```python
from build123d import *

# Parameters (mm, degrees)
BOSS_EXTRUDE1_DEPTH = 1.5
SKETCH2_W           = 77.5
SKETCH2_H           = 28.5
SKETCH2_W_2         = 74.5
SKETCH2_H_2         = 25.5
BOSS_EXTRUDE2_DEPTH = 1.5


with BuildPart() as part:
    # Sketch1 → Boss-Extrude1 (new body)
    with BuildSketch(Plane(origin=(0, 0, 0), x_dir=(1, 0, 0), z_dir=(0, 1, 0))):
        with BuildLine():
            Line((-76.546897521, -86.290788706), (-153.546897521, -86.290788706))
            ThreePointArc((-153.546897521, -86.290788706), (-154.961111084, -85.705002268), (-155.546897521, -84.290788706))
            Line((-155.546897521, -84.290788706), (-155.546897521, -56.290788706))
            ThreePointArc((-155.546897521, -56.290788706), (-154.961111084, -54.876575144), (-153.546897521, -54.290788706))
            Line((-153.546897521, -54.290788706), (-76.546897521, -54.290788706))
            ThreePointArc((-76.546897521, -54.290788706), (-75.132683959, -54.876575144), (-74.546897521, -56.290788706))
            Line((-74.546897521, -56.290788706), (-74.546897521, -84.290788706))
            ThreePointArc((-74.546897521, -84.290788706), (-75.132683959, -85.705002268), (-76.546897521, -86.290788706))
        make_face()
    extrude(amount=BOSS_EXTRUDE1_DEPTH)

    # Sketch2 → Boss-Extrude2 (add)
    with BuildSketch(Plane(origin=(0, 1.5, 0), x_dir=(1, 0, 0), z_dir=(0, 1, 0))):
        with Locations((-115.046897521, -70.290788706)):
            Rectangle(SKETCH2_W, SKETCH2_H)
        with Locations((-115.046897521, -70.290788706)):
            Rectangle(SKETCH2_W_2, SKETCH2_H_2, mode=Mode.SUBTRACT)
    extrude(amount=BOSS_EXTRUDE2_DEPTH)


solid = part.part
```
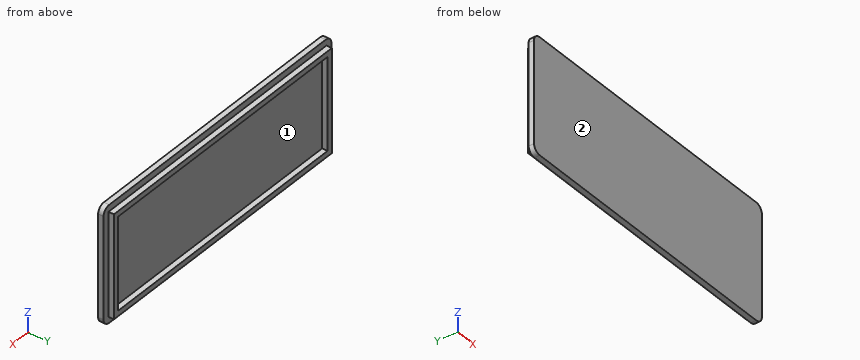
Design review of the part built by this model. Coordinates are the model's own, in mm. Face numbers are marked on the shaded views. Give positions to 0.01 mm unless a question says otherwise; leave off trailing zeros. Loops run counter-clockwise (first coordinate to the right, second up) from the corner with the lowest first, then second, coordinate; pieces in that order, holes last. Notation, with made-up numbers: M 54,-39 L 98,-39 A20 ccw 98,-30 Z; hole C 81.5,65.25 d4. An arc over 180 degrees is marked long. Return JSON: item names as keys, results as strings. Group by question number.
Item 1: We need section B-B (y = 2). Give the boundary of the cut face in (x, z), and give its area (3 significant figures).
Item 2: We need section A-A (x = -132.5). Give the boundary of the cut face in (y, z), and give its area (3 significant figures).
Item 3: For probe 1 along X at (y, z) = (2, 69.5); probe 2 along Z at (x, y) = (-92, 1.65); probe 3 along Y at (x, z) = (-79, 75.5), list the stretches that pass through material, from the lowest coordinate up.
Item 4: Mouldability with a two-part tool opening along X and no side actions: class the marked faces 1 and 2 as released by +X, released by -X, zero draft, split by the parting line, or undercut.
Item 5: We need section C-C (z = 76.5). Give the boundary of the cut face in (x, y), and give its area (3 significant figures).
Item 6: Insertion check: pin 1 Ø1.2 at (y, z) = (2, 65) entering from +X; pin 2 Ø9.5 at (x, z) = (-130.5, 64.5) entering from +Y; pin 3 Ø0.8 at (x, y) = (-113.5, 2) entering from +Z; pin 4 Ø0.8 at (y, z) = (2.5, 71) entering from +X. Each pin has a flat end and moves straight along its axis. Give the tip position at first contact, or say it passes through.
Output:
{
 "1": {"outline": "M -153.8,56.04 L -76.3,56.04 L -76.3,84.54 L -153.8,84.54 Z; hole M -152.3,57.54 L -77.8,57.54 L -77.8,83.04 L -152.3,83.04 Z", "area": "309 mm^2"},
 "2": {"outline": "M 0,54.29 L 1.5,54.29 L 1.5,56.04 L 3,56.04 L 3,57.54 L 1.5,57.54 L 1.5,83.04 L 3,83.04 L 3,84.54 L 1.5,84.54 L 1.5,86.29 L 0,86.29 Z", "area": "52.5 mm^2"},
 "3": {"probe 1": "x = -153.8 to -152.3, -77.8 to -76.3", "probe 2": "z = 56.04 to 57.54, 83.04 to 84.54", "probe 3": "y = 0 to 1.5"},
 "4": {"face 1": "undercut", "face 2": "zero draft"},
 "5": {"outline": "M -155.55,0 L -74.55,0 L -74.55,1.5 L -76.3,1.5 L -76.3,3 L -77.8,3 L -77.8,1.5 L -152.3,1.5 L -152.3,3 L -153.8,3 L -153.8,1.5 L -155.55,1.5 Z", "area": "126 mm^2"},
 "6": {"pin 1": "stops at x = -74.55", "pin 2": "stops at y = 1.5", "pin 3": "stops at z = 84.54", "pin 4": "stops at x = -76.3"}
}
